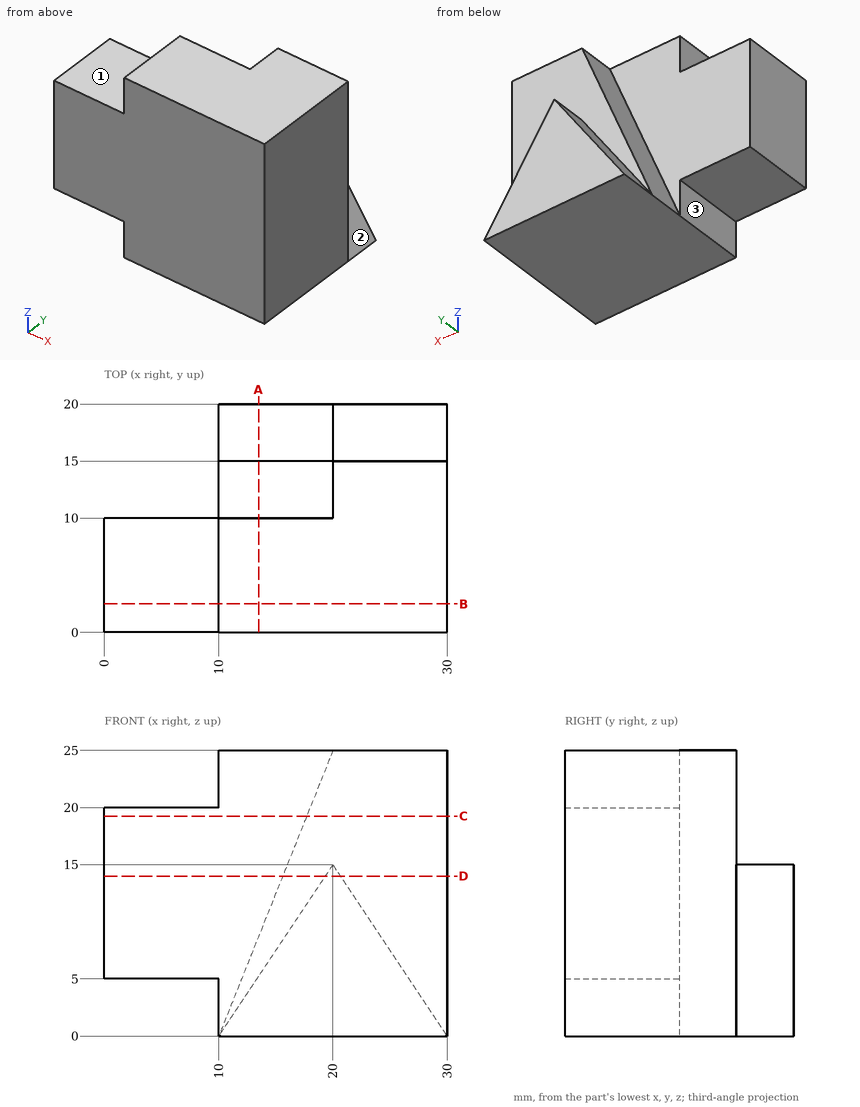
Geometry: see drawing. Coordinates: mm, zero at the bounding-box minimum. A direction names the side the tool comes from. Round coordinates to 2 decimals unless told otherwise and drop trailing zeros. Write each loop counter-clockwise with the first axis right and the second up, starting at its lowest first coordinate (ties: lowest second). Pieces come first, ordered by that corner, then holes. Notation, with made-up numbers: M 52.5,20.5 L 81.5,20.5 A28 cw 81.5,47.5 Z; hole C 32,36.5 d1. An arc over 180 degrees is marked long. Answer as a JSON object with one key per item and string values. Group by question number.
(1) First-contact query: pin 1 (1.5 mm diameter, centred on y = 7, z = 1.5, fed in from -X); pin 2 (8 mm diameter, centred on x = 5, y = 5, fed in from +Z); pin 3 (11 mm diameter, centred on x = 4, y = 5, fed in from -Z). Flat tips, straight axial feed; report the tip coordinate or a pass-through.
(2) Section query D-D on z = 14. Output: boundary loops of the cut face in (x, y), then the cut area to 3 significant figures.
(3) Ray query, line 1 (X direction, y = 4, z = 3.75); line 2 (Z direction, x = 5.5, y = 1.5); line 3 (Y direction, x = 1.5, z = 15). Return the intervals inside material, ascending. Write a range as [from, to].
(4) Section query A-A on x = 13.5. Output: boundary loops of the cut face in (y, z).
(5) Section query B-B on y = 2.5. Output: boundary loops of the cut face in (x, z).
(6) Reachability of the marked faces 1, 2 and 3 from +Z, -Z, +X, -X, +Y, -Y: full face, straight path, thin tool, end or side. Return the list, or none.
(7) Section query C-C on z = 19.25. Output: boundary loops of the cut face in (x, y).
Computed values:
{
 "1": {"pin 1": "x = 10", "pin 2": "z = 20", "pin 3": "z = 5"},
 "2": {"outline": "M 0,0 L 30,0 L 30,15 L 20.67,15 L 20.67,20 L 19.33,20 L 19.33,15 L 15.6,15 L 15.6,10 L 0,10 Z", "area": "379 mm^2"},
 "3": {"line 1": "[10, 30]", "line 2": "[5, 20]", "line 3": "[0, 10]"},
 "4": {"outline": "M 0,0 L 20,0 L 20,5.25 L 15,5.25 L 15,8.75 L 10,8.75 L 10,25 L 0,25 Z"},
 "5": {"outline": "M 0,5 L 10,5 L 10,0 L 30,0 L 30,25 L 10,25 L 10,20 L 0,20 Z"},
 "6": {"face 1": "+Z, -X, +Y, -Y", "face 2": "+Z, +X, +Y", "face 3": "-Z, -X, +Y, -Y"},
 "7": {"outline": "M 0,0 L 30,0 L 30,15 L 17.7,15 L 17.7,10 L 0,10 Z"}
}
